from build123d import *

# Parameters (mm, degrees)
SKETCH1_W                = 78.9
SKETCH1_H                = 4
BOSS_EXTRUDE1_DEPTH      = 76.2
SKETCH2_W                = 46.5
SKETCH2_H                = 26.89406393
BOSS_EXTRUDE2_DEPTH      = 4
SKETCH5_W                = 9.285994966
SKETCH5_H                = 11.707020407
CUT_EXTRUDE2_DEPTH       = 5
SKETCH6_R                = 1.25
CUT_EXTRUDE3_DEPTH       = 85
SKETCH7_W                = 10
SKETCH7_H                = 14
CUT_EXTRUDE4_DEPTH       = 10
SKETCH8_W                = 10
SKETCH8_H                = 14
CUT_EXTRUDE5_DEPTH       = 10
SKETCH9_W                = 3.7
SKETCH9_H                = 45
BOSS_EXTRUDE4_DEPTH      = 56.2
SKETCH10_W               = 46.5
SKETCH10_H               = 8.496116432
BOSS_EXTRUDE5_DEPTH      = 4
SKETCH11_W               = 6.644809846
SKETCH11_H               = 4.508222244
SKETCH11_W_2             = 6.5
BOSS_EXTRUDE6_DEPTH      = 19
SKETCH12_R               = 1.8
CUT_EXTRUDE6_DEPTH       = 19
SKETCH14_R               = 2.3
CUT_EXTRUDE7_DEPTH       = 10
BOSS_EXTRUDE7_DEPTH      = 5
SKETCH16_R               = 1.8
CUT_EXTRUDE8_DEPTH       = 10
BOSS_EXTRUDE8_DEPTH      = 21
BOSS_EXTRUDE9_DEPTH      = 5
CUT_EXTRUDE9_DEPTH       = 5
CUT_EXTRUDE10_DEPTH      = 25
CUT_EXTRUDE10_DEPTH_BACK = 25


with BuildPart() as part:
    # Sketch1 → Boss-Extrude1 (new body)
    with BuildSketch(Plane(origin=(0, 0, 0), x_dir=(1, 0, 0), z_dir=(0, 1, 0))):
        with Locations((39.45, 2)):
            Rectangle(SKETCH1_W, SKETCH1_H)
        Polygon((78.9, 4), (78.9, 0), (78.9, -10), (88.9, -10), (88.9, 4), align=None)
    extrude(amount=BOSS_EXTRUDE1_DEPTH)

    # Sketch2 → Boss-Extrude2 (add)
    with BuildSketch(Plane(origin=(0, 0, -4), x_dir=(-1, 0, 0), z_dir=(0, 0, -1))):
        with Locations((23.25, 13.447031965)):
            Rectangle(SKETCH2_W, SKETCH2_H)
    extrude(amount=-BOSS_EXTRUDE2_DEPTH)

    # Sketch5 → Cut-Extrude2 (cut)
    with BuildSketch(Plane(origin=(0, 0, -4), x_dir=(-1, 0, 0), z_dir=(0, 0, -1))):
        with Locations((-4.642997483, 48.187124879)):
            Rectangle(SKETCH5_W, SKETCH5_H)
    extrude(amount=-CUT_EXTRUDE2_DEPTH, mode=Mode.SUBTRACT)

    # Sketch6 → Cut-Extrude3 (cut)
    with BuildSketch(Plane(origin=(0, 0, 0), x_dir=(-1, 0, 0), z_dir=(0, -1, 0))):
        with Locations(Location((-83.868179675, -5.5, 0), (0, 0, 90))):
            Circle(SKETCH6_R)
    extrude(amount=-CUT_EXTRUDE3_DEPTH, mode=Mode.SUBTRACT)

    # Sketch7 → Cut-Extrude4 (cut)
    with BuildSketch(Plane.XZ):
        with Locations((83.9, 3)):
            Rectangle(SKETCH7_W, SKETCH7_H)
    extrude(amount=-CUT_EXTRUDE4_DEPTH, mode=Mode.SUBTRACT)

    # Sketch8 → Cut-Extrude5 (cut)
    with BuildSketch(Plane(origin=(0, 76.2, 0), x_dir=(1, 0, 0), z_dir=(0, 1, 0))):
        with Locations((83.9, -3)):
            Rectangle(SKETCH8_W, SKETCH8_H)
    extrude(amount=-CUT_EXTRUDE5_DEPTH, mode=Mode.SUBTRACT)

    # Sketch9 → Boss-Extrude4 (add)
    with BuildSketch(Plane(origin=(0, 66.2, 0), x_dir=(1, 0, 0), z_dir=(0, 1, 0))):
        with Locations((88.05, -18.5)):
            Rectangle(SKETCH9_W, SKETCH9_H)
    extrude(amount=-BOSS_EXTRUDE4_DEPTH)

    # Sketch10 → Boss-Extrude5 (add)
    with BuildSketch(Plane.XY):
        with Locations((-23.25, 31.142122146)):
            Rectangle(SKETCH10_W, SKETCH10_H)
    extrude(amount=-BOSS_EXTRUDE5_DEPTH)

    # Sketch11 → Boss-Extrude6 (add)
    with BuildSketch(Plane(origin=(0, 0, -4), x_dir=(-1, 0, 0), z_dir=(0, 0, -1))):
        with Locations((-3.622404923, 24.725888878)):
            Rectangle(SKETCH11_W, SKETCH11_H)
        with Locations((43.25, 24.725888878)):
            Rectangle(SKETCH11_W_2, SKETCH11_H)
    extrude(amount=BOSS_EXTRUDE6_DEPTH)

    # Sketch12 → Cut-Extrude6 (cut)
    with BuildSketch(Plane(origin=(0, 26.98, 0), x_dir=(1, 0, 0), z_dir=(0, 1, 0))):
        with Locations(Location((-44.15, 18.95, 0), (0, 0, 270))):
            Circle(SKETCH12_R)
        with Locations(Location((-44.15, 9.05, 0), (0, 0, 270))):
            Circle(SKETCH12_R)
        with Locations(Location((3.85, 18.95, 0), (0, 0, 270))):
            Circle(SKETCH12_R)
        with Locations(Location((3.85, 9.05, 0), (0, 0, 270))):
            Circle(SKETCH12_R)
    extrude(amount=-CUT_EXTRUDE6_DEPTH, mode=Mode.SUBTRACT)

    # Sketch14 → Cut-Extrude7 (cut)
    with BuildSketch(Plane(origin=(89.9, 0, 0), x_dir=(0, 0, -1), z_dir=(1, 0, 0))):
        with Locations((-36, 37.2)):
            Circle(SKETCH14_R)
    extrude(amount=-CUT_EXTRUDE7_DEPTH, mode=Mode.SUBTRACT)

    # Sketch15 → Boss-Extrude7 (add)
    with BuildSketch(Plane(origin=(0, 35, 0), x_dir=(-1, 0, 0), z_dir=(0, -1, 0))):
        with BuildLine():
            Line((-89.9, -16), (-89.9, 4))
            Line((-89.9, 4), (-167.391867849, -2.779659952))
            ThreePointArc((-167.391867849, -2.779659952), (-160.320800037, -5.70859214), (-157.391867849, -12.779659952))
            ThreePointArc((-157.391867849, -12.779659952), (-159.731423417, -19.207536049), (-165.655386072, -22.627737482))
            Line((-165.655386072, -22.627737482), (-89.9, -16))
        make_face()
        with BuildLine():
            ThreePointArc((-157.391867849, -12.779659952), (-160.320800037, -5.70859214), (-167.391867849, -2.779659952))
            Line((-167.391867849, -2.779659952), (-167.391867849, -22.779659952))
            Line((-167.391867849, -22.779659952), (-165.655386072, -22.627737482))
            ThreePointArc((-165.655386072, -22.627737482), (-159.731423417, -19.207536049), (-157.391867849, -12.779659952))
        make_face()
        with BuildLine():
            Line((-167.391867849, -22.779659952), (-167.391867849, -2.779659952))
            ThreePointArc((-167.391867849, -2.779659952), (-177.391867849, -12.779659952), (-167.391867849, -22.779659952))
        make_face()
    extrude(amount=BOSS_EXTRUDE7_DEPTH)

    # Sketch16 → Cut-Extrude8 (cut)
    with BuildSketch(Plane(origin=(0, 35, 0), x_dir=(1, 0, 0), z_dir=(0, 1, 0))):
        with Locations(Location((167.391867849, -12.779659952, 0), (0, 0, 270))):
            Circle(SKETCH16_R)
        with Locations(Location((143.856470685, -10.758777884, 0), (0, 0, 270))):
            Circle(SKETCH16_R)
    extrude(amount=-CUT_EXTRUDE8_DEPTH, mode=Mode.SUBTRACT)

    # Sketch17 → Boss-Extrude8 (add)
    with BuildSketch(Plane(origin=(0, 0, -4), x_dir=(-1, 0, 0), z_dir=(0, 0, -1))):
        Polygon((-89.9, 44.969099487), (-102.570211114, 35), (-102.570211114, 30), (-89.9, 18.896815366), align=None)
    extrude(amount=-BOSS_EXTRUDE8_DEPTH)

    # Sketch18 → Boss-Extrude9 (add)
    with BuildSketch(Plane(origin=(0, 35, 0), x_dir=(1, 0, 0), z_dir=(0, 1, 0))):
        Polygon((68.155607363, 4), (102.310564972, 6.689173102), (114.279885061, 1.867036439), align=None)
    extrude(amount=-BOSS_EXTRUDE9_DEPTH)

    # Sketch19 → Cut-Extrude9 (cut)
    with BuildSketch(Plane(origin=(0, 35, 0), x_dir=(1, 0, 0), z_dir=(0, 1, 0))):
        with BuildLine():
            Line((167.391867849, -2.779659952), (114.279885061, 1.867036439))
            Line((114.279885061, 1.867036439), (124.22443606, -2.139371913))
            Line((124.22443606, -2.139371913), (143.856470685, -3.758777884))
            ThreePointArc((143.856470685, -3.758777884), (144.565448389, -3.794773963), (145.267134545, -3.902391994))
            Line((145.267134545, -3.902391994), (167.251593152, -6.140542801))
            ThreePointArc((167.251593152, -6.140542801), (168.064444499, -6.173208999), (168.867202147, -6.305021565))
            ThreePointArc((168.867202147, -6.305021565), (172.582949472, -8.638376923), (174.032466733, -12.779659952))
            ThreePointArc((174.032466733, -12.779659952), (172.087480351, -17.475272454), (167.391867849, -19.420258836))
            ThreePointArc((167.391867849, -19.420258836), (166.885463525, -19.400921781), (166.382008444, -19.343023231))
            Line((166.382008444, -19.343023231), (144.811713642, -17.693293793))
            ThreePointArc((144.811713642, -17.693293793), (143.757690083, -17.758080878), (142.705914615, -17.66357482))
            Line((142.705914615, -17.66357482), (102.41543269, -17.09495848))
            Line((102.41543269, -17.09495848), (167.391867849, -22.779659952))
            ThreePointArc((167.391867849, -22.779659952), (177.391867849, -12.779659952), (167.391867849, -2.779659952))
        make_face()
    extrude(amount=-CUT_EXTRUDE9_DEPTH, mode=Mode.SUBTRACT)

    # Sketch21 → Cut-Extrude10 (cut, two sides: drawn at the far end of the back side and taken through both)
    with BuildSketch(Plane(origin=(0, 35, 0), x_dir=(1, 0, 0), z_dir=(0, 1, 0)).offset(-CUT_EXTRUDE10_DEPTH_BACK)):
        Polygon((148.965123629, -18.010952999), (89.9, -13.493561185), (89.9, -22.397972736), align=None)
    extrude(amount=CUT_EXTRUDE10_DEPTH + CUT_EXTRUDE10_DEPTH_BACK, mode=Mode.SUBTRACT)


solid = part.part
Can you work these out from the model? Positions are in its coordinate system, mm. A direction names the side the tool comes from. Round coordinates to 2 decimals unless told otherwise and drop trailing zeros. Loops run counter-clockwise (first coordinate to the right, second up) from the corner with the lowest first, then second, coordinate; pieces in that order, holes last. Notation, with made-up numbers: (74, 62) - (97, 62) arc R23 cw to (97, 87) - close; hole circle Ø2 at (-37.5, -25.5). An arc over 180 degrees is marked (long way). Write item = value, one per line. Start each with the question number.
(1) For faces 1 (the face through (9.286, 48, -2)), 2 (the face through (4, 22.472, -13)), 3 (the face through (4, 26.98, -13)), 4 (the face through (29, 39, 0)), which set-ups out of +Z, -Z, +X, -X, +Y, -Y let a thin tool reach every point of the face, with its end or its side?
(2) If we section it at B-B (y = 63.5): Please give me the cut outline in (x, z), and give its area (3 significant figures).
(3) For P1, Ø5, axis at y = 41, z = 5.5, coming from the -X side; P2, Ø7, axis at x = -42, z = -13.5, coming from the +Y side; P3, Ø8, axis at x = 95.5, z = 9, coming from the -Y side, each with a flat end and sliding along its axis, tell me the tip position at first contact or that it passes through.
(4) If I drill on probe 1 along X at (y, z) = (24.6, -18.95); probe 2 along Z at (x, y) = (87, 37); probe 3 along Z at (x, y) = (33, 6), over which ranges is the centre line in solid material (lowest first)? Write a range as [from, to].
(5) If we section it at C-C (x = -4): Please give me the cut outline in (y, z).
(6) If we section it at A-A (z = 36): Please give me the cut outline in (x, y), and give its area (3 significant figures).
(7) If we section it at D-D (y = 8): Please give me the cut outline in (x, z).
(8) If we mould it in two halves opening along X, with no side actions, what happens to faces 5 (the face through (0, 65, -2)), 6 (the face through (-40, 25, -13)), 7 (the face through (4, 25, -23))? For each: released by +X, released by -X, zero draft, split by the parting line, or undercut.
Ans:
q1.face_1 = +Z, -Z, -X
q1.face_2 = -Z, +X, -X, -Y
q1.face_3 = -Z, +X, -X, +Y
q1.face_4 = +Z, -X, +Y, -Y
q2.outline = (0, -4) - (89.9, -4) - (89.9, 41) - (86.2, 41) - (86.2, 10) - (78.9, 10) - (78.9, 0) - (0, 0) - close; hole circle Ø2.5 at (83.87, 5.5)
q2.area = 579 mm²
q3.P1 = 78.9
q3.P2 = 26.98
q3.P3 = 20.3
q4.probe_1 = [-46.5, -45.95], [-42.35, -40], [0.3, 2.05], [5.65, 6.94]
q4.probe_2 = [-4, 33.71], [38.29, 41]
q4.probe_3 = [-4, 0]
q5.outline = (0, -4) - (35.39, -4) - (35.39, 0) - (0, 0) - close
q6.outline = (86.2, 10) - (89.9, 10) - (89.9, 34.9) - (86.2, 34.9) - close; (86.2, 39.5) - (89.9, 39.5) - (89.9, 66.2) - (86.2, 66.2) - close
q6.area = 191 mm²
q7.outline = (-46.5, -4) - (78.9, -4) - (78.9, 0) - (-46.5, 0) - close
q8.face_5 = released by -X
q8.face_6 = undercut
q8.face_7 = zero draft
